Here's how the part is built. I have some questions about the finished solid (model axes, mm). A direction names the side the tool comes from. Coordinates: 2 decimals unless noted, no trailing zeros. Write each loop counter-clockwise with the first axis right and the second up, starting at its lowest first coordinate (ties: lowest second). Pieces come first, ordered by that corner, then holes. Notation, with made-up numbers: M -24,16.5 L 6,16.5 A17 cw 6,38.5 Z; hole C 77.25,15 d6. An arc over 180 degrees is marked long. Write each question's results on one line, items separated by ' | '. Start each with the question number.
from build123d import *

# Parameters (mm, degrees)
BOSS_EXTRUDE1_DEPTH      = 7.84
SHELL1_START             = -6.87
SHELL1_DEPTH             = 5.9
BOSS_EXTRUDE2_REACH      = 26.75
BOSS_EXTRUDE2_END_RADIUS = 49.03
SKETCH2_R                = 2.45
SKETCH2_R_2              = 1.54
SKETCH3_R                = 2.45
SKETCH3_R_2              = 1.54
BOSS_EXTRUDE3_DEPTH      = 1.8


# Read off the part's stored shape, not the designer's step: Shell1
with BuildPart() as part:
    # Sketch1 → Boss-Extrude1 (new body)
    with BuildSketch(Plane(origin=(0, 0, 0), x_dir=(0, 0, -1), z_dir=(1, 0, 0))):
        with BuildLine():
            Line((22.029982318, -44.885185519), (22.029982318, -43.320185519))
            Line((22.029982318, -43.320185519), (14.149982318, -43.320185519))
            Line((14.149982318, -43.320185519), (14.149982318, -46.450185519))
            Line((14.149982318, -46.450185519), (6.069982318, -46.450185519))
            Line((6.069982318, -46.450185519), (6.069982318, -49.630185519))
            ThreePointArc((6.069982318, -49.630185519), (14.24888625, -47.926706966), (22.029982318, -44.885185519))
        make_face()
    extrude(amount=-BOSS_EXTRUDE1_DEPTH)

    # Shell1 outline → Shell1 (cut)
    with BuildSketch(Plane.YZ.offset(SHELL1_START)):
        with BuildLine():
            Line((-43.320185519, -15.119982318), (-46.640401314, -15.119982318))
            ThreePointArc((-46.640401314, -15.119982318), (-45.555422953, -18.128550399), (-44.276608325, -21.059982318))
            Line((-44.276608325, -21.059982318), (-43.320185519, -21.059982318))
            Line((-43.320185519, -21.059982318), (-43.320185519, -15.119982318))
        make_face()
        with BuildLine():
            Line((-47.420185519, -7.039982318), (-48.521949146, -7.039982318))
            ThreePointArc((-48.521949146, -7.039982318), (-48.047571358, -9.765847969), (-47.420185519, -12.460614163))
            Line((-47.420185519, -12.460614163), (-47.420185519, -7.039982318))
        make_face()
    extrude(amount=SHELL1_DEPTH, mode=Mode.SUBTRACT)

    # Boss-Extrude2: up to this cylinder (the profile starts inside it)
    boss_extrude2_end = Plane(origin=(-3.92, 0, 0), z_dir=(1, 0, 0)) * Cylinder(BOSS_EXTRUDE2_END_RADIUS, 152.56, mode=Mode.PRIVATE)
    # Sketch2 → Boss-Extrude2 (add, up to the surface)
    with BuildSketch(Plane(origin=(0, -41.520185519, 0), x_dir=(1, 0, 0), z_dir=(0, 1, 0)), mode=Mode.PRIVATE) as boss_extrude2_sk1:
        with Locations(Location((-3.92, 18.089982318, 0), (0, 0, 270))):
            Circle(SKETCH2_R)
        with Locations(Location((-3.92, 18.089982318, 0), (0, 0, 270))):
            Circle(SKETCH2_R_2, mode=Mode.SUBTRACT)
    boss_extrude2_tool1 = extrude(boss_extrude2_sk1.sketch, amount=-BOSS_EXTRUDE2_REACH, mode=Mode.PRIVATE) & boss_extrude2_end
    add(boss_extrude2_tool1.solids().sort_by_distance((-3.92, -41.520186, -20.470686))[0])

    # Sketch3 → Boss-Extrude3 (add)
    with BuildSketch(Plane(origin=(0, -46.450185519, 0), x_dir=(1, 0, 0), z_dir=(0, 1, 0))):
        with Locations(Location((-3.92, 10.109982318, 0), (0, 0, 270))):
            Circle(SKETCH3_R)
        with Locations(Location((-3.92, 10.109982318, 0), (0, 0, 270))):
            Circle(SKETCH3_R_2, mode=Mode.SUBTRACT)
    extrude(amount=BOSS_EXTRUDE3_DEPTH)


solid = part.part
1) I want a section at A-A, the plane z = -10. Write out the boundary of the cut face in (x, y).
2) I want a section at D-D, the plane z = -20. Write out the boundary of the cut face in (x, y), then the cut area to 3 significant figures.
3) For faces 1 (the flat face through (-6.87, -48, -9)), 2 (the cylindrical face through (-3.184, -43.41, -15.753)), 3 (the flat face through (-4, -44, -22.03)), which set-ups out of +Z, -Z, +X, -X, +Y, -Y let a thin tool reach every point of the face, with its end or its side?
4) Please list where these lines run through material, in increasing order: line 1 (X direction, y = -44.5, z = -18); line 2 (Z direction, x = -3.92, y = -43.45); line 3 (Z direction, x = -3.92, y = -42.5). Write a range as [from, to].
5) For pin 1 Ø1.5 at (x, z) = (-4.5, -9) entering from +Y; pin 2 Ø2 at (x, z) = (-2, -14.5) entering from -Y; pin 3 Ø4.5 at (x, z) = (-2.5, -10) entering from -Y, each with a flat end and sliding along its axis, tell me the tip position at first contact or that it passes through.
6) I want a section at C-C, the plane y = -42.75. Write out the boundary of the cut face in (x, z).
7) We'd pull the mould along Y, two halves only. Please class faces 4 (the cylindrical face through (-4, -48, -10)), 5 (the cylindrical face through (-2.264, -45.563, -11.916)), 6 (the flat face through (-4, -46.45, -10)): pulls with the +Y half, pulls with the -Y half, needs draft (parallel to the pull), parting line crosses it, or undercut.
8) I want a section at B-B, the plane x = -5.75. Write out the boundary of the cut face in (y, z), then the cut area to 3 significant figures.
Output:
1) outline: M -7.84,-48.99 L 0,-48.99 L 0,-46.45 L -1.47,-46.45 L -1.47,-44.65 L -2.38,-44.65 L -2.38,-46.45 L -5.46,-46.45 L -5.46,-44.65 L -6.37,-44.65 L -6.37,-46.45 L -7.84,-46.45 Z; hole M -6.87,-48 L -0.97,-48 L -0.97,-47.42 L -6.87,-47.42 Z
2) outline: M -7.84,-45.83 L 0,-45.83 L 0,-43.32 L -0.97,-43.32 L -0.97,-44.77 L -2.39,-44.77 L -2.39,-41.52 L -5.45,-41.52 L -5.45,-44.77 L -6.87,-44.77 L -6.87,-43.32 L -7.84,-43.32 Z | area: 21.1 mm2
3) face 1: none | face 2: +Y | face 3: -Z, +X, -X, +Y, -Y
4) line 1: x = [-7.84, -6.87], [-6.37, -5.46], [-2.38, -1.47], [-0.97, 0] | line 2: z = [-22.03, -21.06], [-20.54, -19.63], [-16.55, -15.64], [-15.12, -14.15] | line 3: z = [-20.54, -19.63], [-16.55, -15.64]
5) pin 1: stops at y = -44.65 | pin 2: stops at y = -48.14 | pin 3: stops at y = -49.4
6) outline: C -3.92,-18.09 d4.9; hole C -3.92,-18.09 d3.08
7) face 4: undercut | face 5: needs draft | face 6: pulls with the +Y half
8) outline: M -49.63,-6.07 A50 ccw -44.89,-22.03 L -43.32,-22.03 L -43.32,-21.06 L -44.28,-21.06 A49.03 cw -44.89,-19.72 L -41.52,-19.72 L -41.52,-16.46 L -46.18,-16.46 A49.03 cw -46.64,-15.12 L -43.32,-15.12 L -43.32,-14.15 L -46.45,-14.15 L -46.45,-11.74 L -44.65,-11.74 L -44.65,-8.48 L -46.45,-8.48 L -46.45,-6.07 Z; hole M -48.52,-7.04 A49.03 ccw -47.42,-12.46 L -47.42,-7.04 Z | area: 47.9 mm2
